Geometry check sheet. Reference: the model listing, model coordinates, mm. A direction names the side the tool comes from. Coordinates: 2 decimals unless noted, no trailing zeros. Loops run counter-clockwise (first coordinate to the right, second up) from the corner with the lowest first, then second, coordinate; pieces in that order, holes last.
from build123d import *

# Parameters (mm, degrees)
BOSS_EXTRUDE1_DEPTH  = 20
SKETCH2_R            = 4
CUT_EXTRUDE1_DEPTH   = 17
BOSS_EXTRUDE4_DEPTH  = 17
LPATTERN14_COUNT     = 15
LPATTERN14_PITCH     = 1.6
CUT_EXTRUDE4_DEPTH   = 17
LPATTERN15_COUNT     = 15
LPATTERN15_PITCH     = 1.6
BOSS_EXTRUDE5_DEPTH  = 17
SKETCH10_W           = 2.5
SKETCH10_H           = 16
SKETCH10_W_2         = 3
CUT_EXTRUDE5_DEPTH   = 8.5
CUT_EXTRUDE7_DEPTH   = 16
SKETCH11_4_R         = 4.2
CUT_EXTRUDE8_DEPTH   = 16
CUT_EXTRUDE9_DEPTH   = 16
SKETCH12_3_R         = 4.2
CUT_EXTRUDE10_DEPTH  = 16
SKETCH19_W           = 5
SKETCH19_H           = 40.8
BOSS_EXTRUDE8_DEPTH  = 20
CUT_EXTRUDE11_DEPTH  = 6
SKETCH23_W           = 50
SKETCH23_H           = 4
SKETCH23_H_2         = 9.2
SKETCH23_H_3         = 17.2
CUT_EXTRUDE12_DEPTH  = 106.531796156
CUT_EXTRUDE15_REACH  = 126.828
SKETCH28_W           = 55.4
SKETCH28_H           = 7
BOSS_EXTRUDE10_REACH = 116.365


with BuildPart() as part:
    # Sketch1 → Boss-Extrude1 (new body)
    with BuildSketch(Plane(origin=(0, 0, 0), x_dir=(1, 0, 0), z_dir=(0, 1, 0))):
        Polygon((0, 0), (76.4, 0), (76.4, 16), (76.4, 70), (0, 70), align=None)
    extrude(amount=BOSS_EXTRUDE1_DEPTH)

    # Sketch2 → Cut-Extrude1 (cut)
    with BuildSketch(Plane(origin=(0, 20, 0), x_dir=(1, 0, 0), z_dir=(0, 1, 0))):
        with BuildLine():
            Line((25, 9.4), (25, 0))
            Line((25, 0), (28, 0))
            Line((28, 0), (28, 8.18))
            Line((28, 8.18), (49, 8.18))
            Line((49, 8.18), (49.046786118, 8.18))
            ThreePointArc((49.046786118, 8.18), (49, 8.79), (49.046786118, 9.4))
            Line((49.046786118, 9.4), (49, 9.4))
            Line((49, 9.4), (28, 9.4))
            Line((28, 9.4), (25, 9.4))
        make_face()
        with Locations((53, 8.79)):
            Circle(SKETCH2_R)
    extrude(amount=-CUT_EXTRUDE1_DEPTH, mode=Mode.SUBTRACT)

    # Sketch4 → Boss-Extrude4 (add)
    with BuildSketch(Plane(origin=(0, 20, 0), x_dir=(1, 0, 0), z_dir=(0, 1, 0))):
        with BuildLine():
            Line((25.4, 9.4), (25, 9.4))
            ThreePointArc((25, 9.4), (25.4, 9), (25.8, 9.4))
            Line((25.8, 9.4), (25.4, 9.4))
        make_face()
    boss_extrude4 = extrude(amount=-BOSS_EXTRUDE4_DEPTH)

    # LPattern14: Boss-Extrude4 ×15
    with Locations(*[(i * LPATTERN14_PITCH, 0, 0) for i in range(1, LPATTERN14_COUNT)]):
        add(boss_extrude4)

    # Sketch8 → Cut-Extrude4 (cut)
    with BuildSketch(Plane(origin=(0, 20, 0), x_dir=(1, 0, 0), z_dir=(0, 1, 0))):
        with BuildLine():
            Line((25.8, 9.4), (26.6, 9.4))
            ThreePointArc((26.6, 9.4), (26.2, 9.8), (25.8, 9.4))
        make_face()
    cut_extrude4 = extrude(amount=-CUT_EXTRUDE4_DEPTH, mode=Mode.SUBTRACT)

    # LPattern15: Cut-Extrude4 ×15
    with Locations(*[(i * LPATTERN15_PITCH, 0, 0) for i in range(1, LPATTERN15_COUNT)]):
        add(cut_extrude4, mode=Mode.SUBTRACT)

    # Sketch9 → Boss-Extrude5 (add)
    with BuildSketch(Plane(origin=(0, 20, 0), x_dir=(1, 0, 0), z_dir=(0, 1, 0))):
        Polygon((28, 8.18), (28, 8.34), (48.939227735, 8.34), (49.046786118, 8.34), (49.046786118, 8.18), align=None)
    extrude(amount=-BOSS_EXTRUDE5_DEPTH)

    # Sketch10 → Cut-Extrude5 (cut)
    with BuildSketch(Plane(origin=(0, 20, 0), x_dir=(1, 0, 0), z_dir=(0, 1, 0))):
        with Locations((7.25, 8)):
            Rectangle(SKETCH10_W, SKETCH10_H)
        with Locations((68.9, 8)):
            Rectangle(SKETCH10_W_2, SKETCH10_H)
    extrude(amount=-CUT_EXTRUDE5_DEPTH, mode=Mode.SUBTRACT)

    # Sketch11 → Cut-Extrude7 (cut)
    with BuildSketch(Plane.XY):
        with BuildLine():
            Line((7.25, 11.5), (6, 11.5))
            Line((6, 11.5), (6, 11.309675797))
            ThreePointArc((6, 11.309675797), (6.617796848, 11.452146333), (7.25, 11.5))
        make_face()
        with BuildLine():
            Line((8.5, 11.5), (7.25, 11.5))
            ThreePointArc((7.25, 11.5), (7.882203152, 11.452146333), (8.5, 11.309675797))
            Line((8.5, 11.309675797), (8.5, 11.5))
        make_face()
    extrude(amount=-CUT_EXTRUDE7_DEPTH, mode=Mode.SUBTRACT)

    # Sketch11<4> → Cut-Extrude8 (cut)
    with BuildSketch(Plane.XY):
        with Locations((7.25, 7.3)):
            Circle(SKETCH11_4_R)
    extrude(amount=-CUT_EXTRUDE8_DEPTH, mode=Mode.SUBTRACT)

    # Sketch12 → Cut-Extrude9 (cut)
    with BuildSketch(Plane.XY):
        with BuildLine():
            Line((68.9, 11.5), (67.4, 11.5))
            Line((67.4, 11.5), (67.4, 11.223009049))
            ThreePointArc((67.4, 11.223009049), (68.13731986, 11.430171789), (68.9, 11.5))
        make_face()
        with BuildLine():
            Line((70.4, 11.5), (68.9, 11.5))
            ThreePointArc((68.9, 11.5), (69.66268014, 11.430171789), (70.4, 11.223009049))
            Line((70.4, 11.223009049), (70.4, 11.5))
        make_face()
    extrude(amount=-CUT_EXTRUDE9_DEPTH, mode=Mode.SUBTRACT)

    # Sketch12<3> → Cut-Extrude10 (cut)
    with BuildSketch(Plane.XY):
        with Locations((68.9, 7.3)):
            Circle(SKETCH12_3_R)
    extrude(amount=-CUT_EXTRUDE10_DEPTH, mode=Mode.SUBTRACT)

    # Sketch19 → Boss-Extrude8 (add)
    with BuildSketch(Plane(origin=(0, 20, 0), x_dir=(1, 0, 0), z_dir=(0, 1, 0))):
        Polygon((0, 62.7), (0, 70), (-25, 70), (-25, 62.7), (-20, 62.7), align=None)
        with Locations((-22.5, 42.3)):
            Rectangle(SKETCH19_W, SKETCH19_H)
        Polygon((0, 14.6), (0, 21.9), (-20, 21.9), (-25, 21.9), (-25, 14.6), align=None)
    extrude(amount=-BOSS_EXTRUDE8_DEPTH)

    # Sketch22 → Cut-Extrude11 (cut)
    with BuildSketch(Plane(origin=(0, 20, 0), x_dir=(1, 0, 0), z_dir=(0, 1, 0))):
        Polygon((-25, 14.6), (0, 14.6), (0, 21.9), (-20, 21.9), (-20, 62.7), (0, 62.7), (0, 70), (-25, 70), align=None)
    extrude(amount=-CUT_EXTRUDE11_DEPTH, mode=Mode.SUBTRACT)

    # Sketch23 → Cut-Extrude12 (cut, through all)
    with BuildSketch(Plane(origin=(0, 20, 0), x_dir=(1, 0, 0), z_dir=(0, 1, 0))):
        with Locations((38.2, 63.7)):
            Rectangle(SKETCH23_W, SKETCH23_H)
        with Locations((38.2, 57.1)):
            Rectangle(SKETCH23_W, SKETCH23_H_2)
        with Locations((38.2, 43.9)):
            Rectangle(SKETCH23_W, SKETCH23_H_3)
    extrude(amount=-CUT_EXTRUDE12_DEPTH, mode=Mode.SUBTRACT)

    # Cut-Extrude15: up to this face of the body (flat: up to its plane)
    cut_extrude15_end = Plane(part.part.faces().sort_by_distance((0, 10.512880562, -33.751990632))[0])
    # Sketch28 → Cut-Extrude15 (cut, up to the picked face)
    with BuildSketch(Plane.ZY.offset(25), mode=Mode.PRIVATE) as cut_extrude15_sk1:
        with Locations((-42.3, 10.5)):
            Rectangle(SKETCH28_W, SKETCH28_H)
    cut_extrude15_tool1 = split(extrude(cut_extrude15_sk1.sketch, amount=-CUT_EXTRUDE15_REACH, mode=Mode.PRIVATE), bisect_by=cut_extrude15_end, keep=Keep.BOTH, mode=Mode.PRIVATE)
    add(cut_extrude15_tool1.solids().sort_by(Axis((-25, 10.5, -42.3), (1, 0, 0)))[0], mode=Mode.SUBTRACT)

    # Sketch29 → Boss-Extrude10 (add, up to next)
    with BuildSketch(Plane.ZY.offset(-63.2), mode=Mode.PRIVATE) as boss_extrude10_sk1:
        Polygon((-65.7, 0), (-57.7, 0), (-65.7, 20), align=None)
    boss_extrude10_tool1 = extrude(boss_extrude10_sk1.sketch, amount=BOSS_EXTRUDE10_REACH, mode=Mode.PRIVATE) - part.part
    # Sketch29 → Boss-Extrude10 (add, up to next)
    with BuildSketch(Plane.ZY.offset(-63.2), mode=Mode.PRIVATE) as boss_extrude10_sk2:
        Polygon((-35.3, 0), (-45.3, 0), (-35.3, 20), align=None)
    boss_extrude10_tool2 = extrude(boss_extrude10_sk2.sketch, amount=BOSS_EXTRUDE10_REACH, mode=Mode.PRIVATE) - part.part
    add(boss_extrude10_tool1.solids().sort_by_distance((63.2, 6.666667, -63.033333))[0])
    add(boss_extrude10_tool2.solids().sort_by_distance((63.2, 6.666667, -38.633333))[0])


solid = part.part
1) Material ranges on probe 1 along Z at (x, y) = (53, 13.75) (3 decimals); probe 2 along Z at (x, y) = (53, 16.25) (3 decimals); probe 3 along X at (y, z) = (11.5, -6), recorded low to high.
Data:
probe 1: z = -70 to -63.2, -38.425 to -12.79, -4.79 to 0
probe 2: z = -70 to -64.2, -37.175 to -12.79, -4.79 to 0
probe 3: x = 0 to 6, 8.5 to 25, 28 to 50.13, 55.87 to 67.4, 70.4 to 76.4
2) Section check A-A on x = -13. Record the cut outline in (y, z), and give its area (3 significant figures).
Data:
outline: (0, -70) - (7, -70) - (7, -62.7) - (0, -62.7) - close; (0, -21.9) - (7, -21.9) - (7, -14.6) - (0, -14.6) - close
area: 102 mm2
3) Section check B-B on z = -49. Record the cut outline in (x, y), and give its area (3 significant figures).
Data:
outline: (-25, 0) - (-20, 0) - (-20, 7) - (-25, 7) - close; (0, 0) - (13.2, 0) - (13.2, 20) - (0, 20) - close; (63.2, 0) - (76.4, 0) - (76.4, 20) - (63.2, 20) - close
area: 563 mm2
4) Section check D-D on x = 51.5. Record the cut outline in (y, z), and give its area (3 significant figures).
Data:
outline: (0, -70) - (20, -70) - (20, -65.7) - (0, -57.7) - close; (0, -45.3) - (20, -35.3) - (20, -12.5) - (3, -12.5) - (3, -5.08) - (20, -5.08) - (20, 0) - (0, 0) - close
area: 846 mm2
5) Depth check by flat-ended pin: pin 1 (3.5 mm diameter, centred on x = -12, y = 3.5, fed in from +Z); pin 2 (1 mm diameter, centred on y = 11, z = -27.5, fed in from -X). Enter the tip coordinate at first touch or a pass-through.
Data:
pin 1: stops at z = -14.6
pin 2: stops at x = 0
6) Access from +Z, -Z, +X, -X, +Y, -Y to the whole of each face (thin tool, end or side, straight path). Record for faces 1 (the flat face through (28, 12, -4)), 2 (the flat face through (-20, 4, -42)), 3 (the flat face through (-13, 4, -14.6)), 4 (the cylindrical face through (68.737, 3.103, -7.888)), 5 (the flat face through (38.55, 9.86, -40.37)).
Data:
face 1: +Z, +Y
face 2: +Y, -Y
face 3: +Z, -X, +Y, -Y
face 4: +Z
face 5: +Y
7) Mould release check, pull along X, two halves, no side actions. Record for faces 6 (the flat face through (-21, 7, -43)), 7 (the flat face through (-25, 4, -43)), 8 (the flat face through (0, 10, -35)), 9 (the cylindrical face through (7.083, 3.103, -7.888)): +X half, -X half, draft (parallel to the pull), parting line (faces both ways), or undercut.
Data:
face 6: draft
face 7: -X half
face 8: undercut
face 9: undercut
8) Section check C-C on x = 68.9. Record the cut outline in (y, z).
Data:
outline: (0, -70) - (20, -70) - (20, -16) - (3.1, -16) - (3.1, 0) - (0, 0) - close
